The figure shows three views and two pictorial views of one solid part (mm, origin at its lowest corner). Answer the questions. A direction names the side the tool comes from. Coordinates: 2 decimals unless noted, no trailing zeros. Order: outer loops, then holes, each group sorted by start corner. A loop starts at its lowest first (then second) coordinate and runs counter-clockwise, first axis right, second up. Notation, with made-up numbers: (77.25, 45) -> (121.25, 45) arc R30 ccw to (121.25, 83) -> close; hole circle Ø6 at (61.5, 8). An arc over 180 degrees is marked (long way). Return JSON: item names as keys, results as strings.
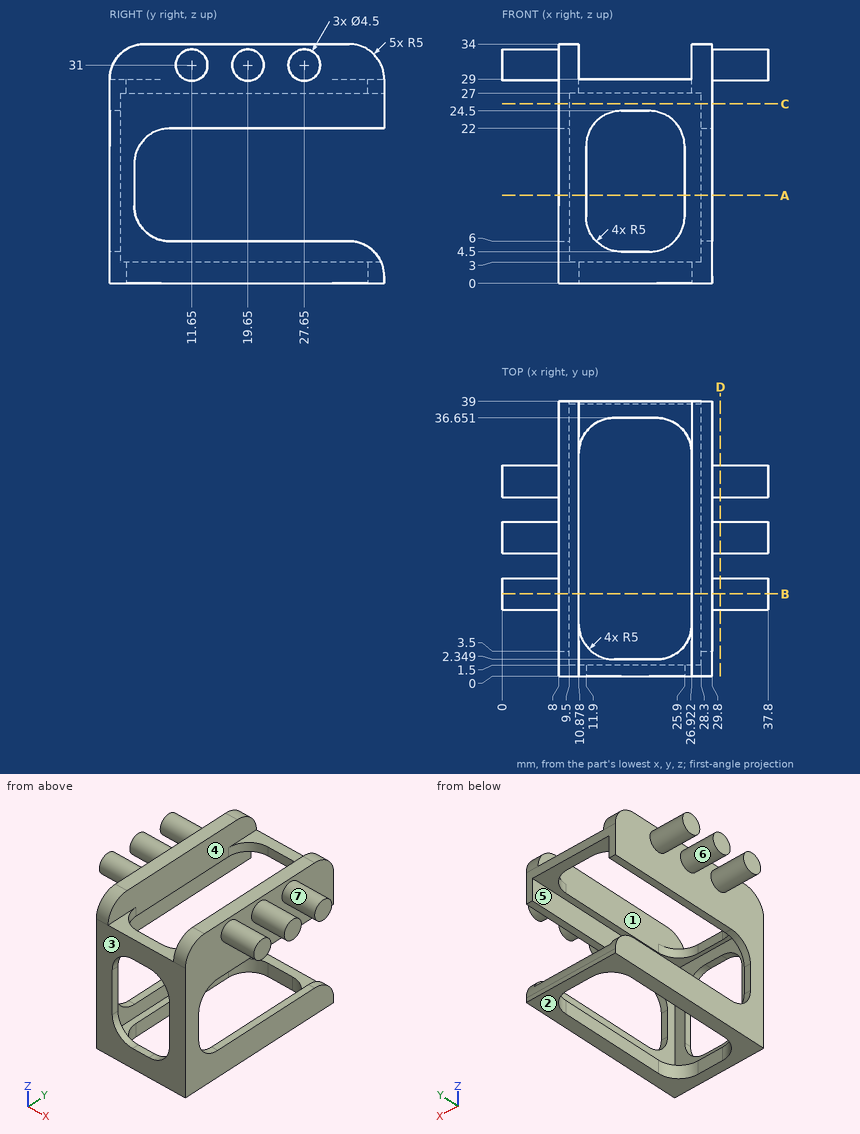
Item 1: Find the intervals of material crossed by probe 1 along X at (y, z) = (17.5, 4.5); probe 2 along Z at (x, y) = (28, 11.5); probe 3 along Z at (x, y) = (8.5, 30.5), in increasing order.
Answer list:
{"probe 1": "8 to 9.5, 28.3 to 29.8", "probe 2": "0 to 3, 27 to 34", "probe 3": "0 to 6, 22 to 34"}
Item 2: The part is cut by section B-B on y = 11.65. Count the separate pieces of the cut face and the enclosed holes in it, plus the area to 3 significant figures.
Answer list:
{"separate pieces": "4", "enclosed holes": "0", "area": "154 mm2"}
Item 3: The part is cut by section A-A on z = 12.5. Determine the outline of the cut face in (x, y), plus the area to 3 significant figures.
Answer list:
{"outline": "(8, 0) -> (11.9, 0) -> (11.9, 1.5) -> (9.5, 1.5) -> (9.5, 3.5) -> (8, 3.5) -> close; (25.9, 0) -> (29.8, 0) -> (29.8, 3.5) -> (28.3, 3.5) -> (28.3, 1.5) -> (25.9, 1.5) -> close", "area": "17.7 mm2"}
Item 4: The part is cut by section D-D on x = 31. Determine the outline of the cut face in (y, z).
Answer list:
{"outline": "circle Ø4.5 at (11.65, 31); circle Ø4.5 at (19.65, 31); circle Ø4.5 at (27.65, 31)"}
Item 5: Which of the six approach directions +Z, -Z, +X, -X, +Y, -Y give full straight-line access (tool end or side, diameter ignored) to the marked faces 4, 5, 6 and 7?
Answer list:
{"face 4": "+Z", "face 5": "+Y", "face 6": "-X", "face 7": "+X"}
Item 6: Flat-ended cylindrical pins translate along their axes: pin 1 (0.9 mm diameter, centred on x = 18, z = 2, fed in from +Y); pin 2 (0.8 mm diameter, centred on x = 19, y = 0.5, fed in from +Z); pin 3 (15 mm diameter, centred on x = 19, y = 21.5, fed in from +Z); pin 4 (19 mm diameter, centred on y = 13, z = 13, fed in from +X). Find the tip coordinate at first contact, or state that the pin passes through.
Answer list:
{"pin 1": "y = 38.97", "pin 2": "z = 29", "pin 3": "through", "pin 4": "x = 29.8"}
Item 7: The part is cut by section C-C on z = 25.5. Determine the outline of the cut face in (x, y), plus the area to 3 significant figures.
Answer list:
{"outline": "(8, 0) -> (29.8, 0) -> (29.8, 39) -> (28.3, 39) -> (28.3, 1.5) -> (9.5, 1.5) -> (9.5, 39) -> (8, 39) -> close", "area": "145 mm2"}
Item 8: Determine the mould class of the marked faces 1, 2 and 3 for opening direction Y: pulls with the +Y half, pulls with the -Y half, needs draft (parallel to the pull), parting line crosses it, or undercut.
Answer list:
{"face 1": "undercut", "face 2": "needs draft", "face 3": "pulls with the -Y half"}
